from build123d import *

# Parameters (mm, degrees)
BOX001_W     = 5.2
BOX001_H     = 5.2
BOX001_DEPTH = 3
BOX003_W     = 5.2
BOX003_H     = 5.2
BOX003_DEPTH = 3
BOX002_W     = 5.2
BOX002_H     = 5.2
BOX002_DEPTH = 3
BOX_W        = 20
BOX_H        = 20
BOX_DEPTH    = 2.5
FILLET_R     = 1
FILLET001_R  = 1


with BuildPart() as obj1:
    # Box001 → Box001 (new body)
    with BuildSketch(Plane(origin=(7.4, 0, 1.5), x_dir=(1, 0, 0), z_dir=(0, 0, 1))):
        with Locations((2.6, 2.6)):
            Rectangle(BOX001_W, BOX001_H)
    extrude(amount=BOX001_DEPTH)


with BuildPart() as obj2:
    # Box003 → Box003 (new body)
    with BuildSketch(Plane(origin=(0, 7.4, 1.5), x_dir=(1, 0, 0), z_dir=(0, 0, 1))):
        with Locations((2.6, 2.6)):
            Rectangle(BOX003_W, BOX003_H)
    extrude(amount=BOX003_DEPTH)


with BuildPart() as obj3:
    # Box002 → Box002 (new body)
    with BuildSketch(Plane(origin=(7.4, 14.8, 1.5), x_dir=(1, 0, 0), z_dir=(0, 0, 1))):
        with Locations((2.6, 2.6)):
            Rectangle(BOX002_W, BOX002_H)
    extrude(amount=BOX002_DEPTH)


with BuildPart() as fusion:
    # Box → Box (new body)
    with BuildSketch(Plane.XY):
        with Locations((10, 10)):
            Rectangle(BOX_W, BOX_H)
    extrude(amount=BOX_DEPTH)

    # Fillet
    fillet_edges = [fusion.edges().sort_by_distance(p)[0] for p in [
        (0, 0, 1.25),
        (0, 20, 1.25),
        (20, 0, 1.25),
        (20, 20, 1.25),
    ]]
    fillet(fillet_edges, radius=FILLET_R)

    # Fillet001
    fillet001_edges = [fusion.edges().sort_by_distance(p)[0] for p in [
        (0, 10, 0),
        (0.292893, 0.292893, 0),
        (0.292893, 19.707107, 0),
        (10, 0, 0),
        (10, 20, 0),
        (19.707107, 0.292893, 0),
        (19.707107, 19.707107, 0),
        (20, 10, 0),
    ]]
    fillet(fillet001_edges, radius=FILLET001_R)

    # Fusion: union obj1, obj2, obj3
    add(obj1.part)
    add(obj2.part)
    add(obj3.part)


solid = fusion.part
Can you work these out from the model? Positions are in its coordinate system, mm. A direction names the side the tool comes from. Coordinates: 2 decimals unless noted, no trailing zeros. Write each loop counter-clockwise with the first axis right and the second up, starting at its lowest first coordinate (ties: lowest second). Pieces come first, ordered by that corner, then holes. Notation, with made-up numbers: (21, -26.75) -> (29, -26.75) arc R19 cw to (29, -10.75) -> close; hole circle Ø8 at (77.5, 3). An arc over 180 degrees is marked (long way). Write each question's results on one line, items separated by ' | '. Start each with the question number.
Item 1: If we section it at A-A, the plane z = 3.75: Write out the boundary of the cut face in (x, y).
Item 2: I'm going to push flat-ended pins straight in: P1, Ø0.6, axis at x = 3, z = 3, coming from the -Y side; P2, Ø0.6, axis at y = 3.5, z = 3.5, coming from the +X side; P3, Ø1, axis at x = 2.5, z = 3.5, coming from the +Y side. Where does each tip first touch, or does it pass through?
Item 3: If we section it at D-D, the plane z = 0.4: Write out the boundary of the cut face in (x, y), and give its area (3 significant figures).
Item 4: Thinking about a two-plate mould opening in Y: for faces 1 (the flat face through (10, 5.2, 3)), 2 (the flat face through (12.6, 3, 3)), 3 (the cylindrical face through (19.699, 0.285, 1.76)), which applies, released by +Y, released by -Y, zero draft, split by the parting line, or undercut?
Item 5: If we section it at B-B, the plane x = 9.5: Write out the boundary of the cut face in (y, z).
Item 6: On a 3-axis mill with a long thin cutter (end or side, diameter ignored), from which of +Z, -Z, +X, -X, +Y, -Y can I reach the whole of each face in a straight line? I mean faces 4 (the cylindrical face through (19.715, 19.699, 1.76)), 5 (the flat face through (12.6, 17, 3)), 6 (the flat face through (3, 12.6, 3)). Say none if no direction works.
Item 7: Please list where these lines run through material, in increasing order: probe 1 along Z at (x, y) = (1.75, 1.25); probe 2 along X at (y, z) = (18.25, 3.4); probe 3 along Y at (x, z) = (4.5, 0.95).
Item 8: If we section it at C-C, the plane y = 18.75: Write out the boundary of the cut face in (x, z), and give its area (3 significant figures).
Answer block:
1) outline: (0, 7.4) -> (5.2, 7.4) -> (5.2, 12.6) -> (0, 12.6) -> close; (7.4, 0) -> (12.6, 0) -> (12.6, 5.2) -> (7.4, 5.2) -> close; (7.4, 14.8) -> (12.6, 14.8) -> (12.6, 20) -> (7.4, 20) -> close
2) P1: y = 7.4 | P2: x = 12.6 | P3: y = 12.6
3) outline: (0.2, 1) arc R0.8 ccw to (1, 0.2) -> (19, 0.2) arc R0.8 ccw to (19.8, 1) -> (19.8, 19) arc R0.8 ccw to (19, 19.8) -> (1, 19.8) arc R0.8 ccw to (0.2, 19) -> close | area: 384 mm²
4) face 1: undercut | face 2: zero draft | face 3: released by -Y
5) outline: (0, 1) arc R1 ccw to (1, 0) -> (19, 0) arc R1 ccw to (20, 1) -> (20, 4.5) -> (14.8, 4.5) -> (14.8, 2.5) -> (5.2, 2.5) -> (5.2, 4.5) -> (0, 4.5) -> close
6) face 4: +Z, -Z, +X, +Y | face 5: +Z, +X, +Y, -Y | face 6: +Z, +X, -X, +Y
7) probe 1: 0 to 2.5 | probe 2: 7.4 to 12.6 | probe 3: 0 to 20
8) outline: (0, 1) arc R1 ccw to (1, 0) -> (19, 0) arc R1 ccw to (20, 1) -> (20, 2.5) -> (12.6, 2.5) -> (12.6, 4.5) -> (7.4, 4.5) -> (7.4, 2.5) -> (0, 2.5) -> close | area: 60.0 mm²
